Verification items for the finished model (mm, model axes). Round coordinates to 2 decimals unless told otherwise and drop trailing zeros. Write each loop counter-clockwise with the first axis right and the second up, starting at its lowest first coordinate (ties: lowest second). Pieces come first, ordered by that corner, then holes. Notation, with made-up numbers: (3, 67) -> (25, 67) arc R21 cw to (25, 86) -> close; hole circle Ø4 at (-4, -10). An arc over 180 degrees is marked (long way). Answer as a JSON object with one key per item and string values. Group by question number.
(1) Scan lines: L1, parallel to Y at x = 0, z = 14.05; L2, parallel to X at y = 27.94, z = 12.6; L3, parallel to Y at x = 2.25, z = 14.75. Record each from-to range of solid material in increasing order. Write a range as from..to.
(2) Draft check along X on faces 1 (the face through (2.288, 15.027, 11.751)), 2 (the face through (-0.06, 29.21, 12.67)), 3 (the face through (-0.9, 0, 15.2)). Enter one of: released by +X, released by -X, zero draft, split by the parting line, or undercut.
(3) Gauge pin test, flat ends, axial feed: pin 1 Ø4 at (x, y) = (0, 27.94) entering from -Z; pin 2 Ø4 at (x, y) = (-1, 4.5) entering from +Z; pin 3 Ø2 at (x, y) = (-2, 13) entering from -Z. Record the tip position at first contact, or that the pin passes through.
(4) Sectioned sample at A-A on x = 0.75. Record the cut outline in (y, z).
(5) Sectioned sample at D-D on x = -0.5. Record the cut outline in (y, z).
(6) Sectioned sample at B-B on y = 27.94. Record the cut outline in (x, z), and give its area (3 significant figures).
(7) Sectioned sample at C-C on z = 12. Record the cut outline in (x, y).
Autodesk Fusion 360 part; units mm, degrees
sketch "Sketch1" plane through (0, 0, 0) normal (0, 1, 0) x (1, 0, 0)
  circle A0 centre (0, -12.7) radius 2.4765
  dimension "d1" = 4.953
extrude "Extrude1" add sketch "Sketch1" along normal blind 30.48
hole "Hole1" at (0, 27.94, 15.1765) direction (0, 0, -1) diameter 2.54 depth 10.668 tip angle 118
sketch "Sketch2" plane through (0, 0, 0) normal (0, -1, 0) x (1, 0, 0)
  circle A0 centre (0, 12.7) radius 2.4765
  line L0 (-1.27, 11.43) -> (1.27, 11.43)
  line L1 (1.27, 11.43) -> (1.27, 13.97)
  line L2 (1.27, 13.97) -> (-1.27, 13.97)
  line L3 (-1.27, 13.97) -> (-1.27, 11.43)
extrude "Extrude2" add sketch "Sketch2" along normal blind 2.54 contours L0 L1 L2 L3
extrude "Extrude3" add 1 faces at (0.4233, -0.8467, 13.97) along direction (0, 0, 1) blind 2.54
extrude "Extrude4" add 1 faces at (-0.4233, -0.8467, 11.43) along direction (0, 0, -1) blind 2.54
extrude "Extrude5" add 1 faces at (-1.27, -1.6933, 11.9913) along direction (-1, 0, 0) blind 2.54
extrude "Extrude6" add 1 faces at (1.27, -1.6933, 11.9913) along direction (1, 0, 0) blind 2.54
fillet "Fillet1" radius 3.81 4 edges at (-3.81, -1.27, 16.51) (3.81, -1.27, 16.51) (3.81, -1.27, 8.89) (-3.81, -1.27, 8.89)
Computed values:
{
 "1": {"L1": "-2.54..26.67, 29.21..30.48", "L2": "-2.47..-1.27, 1.27..2.47", "L3": "-2.54..0"},
 "2": {"face 1": "split by the parting line", "face 2": "undercut", "face 3": "zero draft"},
 "3": {"pin 1": "z = 10.22", "pin 2": "z = 15.18", "pin 3": "z = 10.43"},
 "4": {"outline": "(-2.54, 8.96) -> (0, 8.96) -> (0, 10.34) -> (26.92, 10.34) -> (26.92, 15.06) -> (0, 15.06) -> (0, 16.44) -> (-2.54, 16.44) -> close; (28.96, 10.34) -> (30.48, 10.34) -> (30.48, 15.06) -> (28.96, 15.06) -> close"},
 "5": {"outline": "(-2.54, 8.92) -> (0, 8.92) -> (0, 10.27) -> (26.77, 10.27) -> (26.77, 15.13) -> (0, 15.13) -> (0, 16.48) -> (-2.54, 16.48) -> close; (29.11, 10.27) -> (30.48, 10.27) -> (30.48, 15.13) -> (29.11, 15.13) -> close"},
 "6": {"outline": "(-1.27, 10.57) -> (-1.27, 14.83) arc R2.48 ccw to start; (1.27, 10.57) arc R2.48 ccw to (1.27, 14.83) -> close", "area": "7.26 mm2"},
 "7": {"outline": "(-3.75, -2.54) -> (3.75, -2.54) -> (3.75, 0) -> (2.38, 0) -> (2.38, 30.48) -> (-2.38, 30.48) -> (-2.38, 0) -> (-3.75, 0) -> close; hole circle Ø2.54 at (0, 27.94)"}
}
